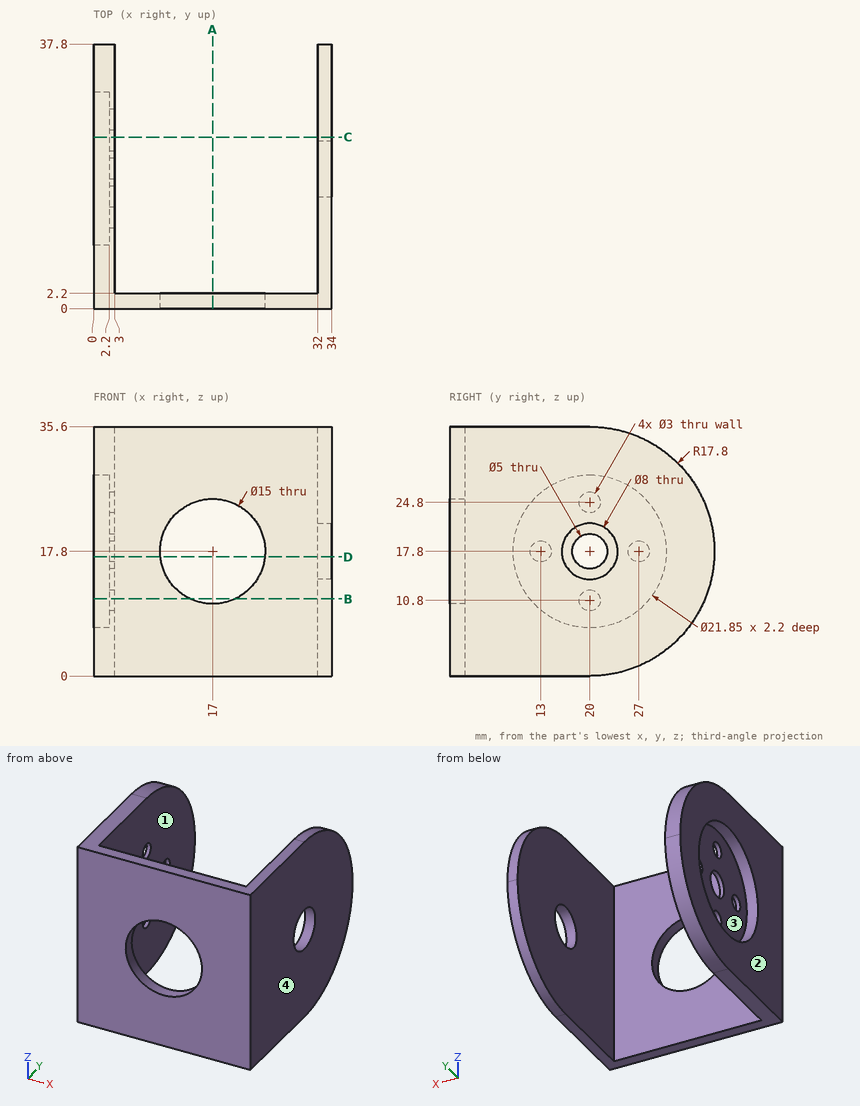
The figure shows three views and two pictorial views of one solid part (mm, origin at its lowest corner). Answer the questions. A direction names the side the tool comes from. Coordinates: 2 decimals unless noted, no trailing zeros. Loops run counter-clockwise (first coordinate to the right, second up) from the corner with the lowest first, then second, coordinate; pieces in that order, holes last. Notation, with made-up numbers: (25.25, 64.5) -> (73.25, 64.5) arc R22 ccw to (73.25, 96.5) -> close; hole circle Ø4 at (78.25, 65). An arc over 180 degrees is marked (long way). Return JSON: item names as keys, results as strings. Group by question number.
(1) Given pin 1 Ø3.5 at (y, z) = (27, 17.8) entering from -X; pin 2 Ø2.5 at (y, z) = (20, 10.8) entering from -X; pin 3 Ø7 at (y, z) = (20, 17.8) entering from +X; pin 4 Ø10 at (x, y) = (25, 22.5) entering from -Z, each flat-ended and moving along its own axis, determine where each tip first touches the part or whether it passes through.
(2) A cutting plane is placed at C-C on y = 24.5. Write down the section's boundary in (x, z).
(3) A cutting plane is placed at D-D on z = 17. Count the separate pieces of the cut face and the enclosed holes in it, and give its area (3 significant figures).
(4) Find the intervals of material crossed by probe 1 along X at (y, z) = (28, 7); probe 2 along Y at (x, z) = (32.6, 17.8); probe 3 along X at (y, z) = (28.5, 16.5), in increasing order. Write a range as from..to.
(5) A cutting plane is placed at B-B on z = 11. Write down the section's boundary in (x, y).
(6) Determine the mould class of the marked faces 3 and 4 for opening direction Z: released by +Z, released by -Z, zero draft, split by the parting line, or undercut.
(7) A cutting plane is placed at A-A on x = 17. Write down the section's boundary in (y, z), and give its area (3 significant figures).
(8) Which of the six approach directions +Z, -Z, +X, -X, +Y, -Y give full straight-line access (tool end or side, diameter ignored) to the marked faces 1 and 2?
The answers:
{
 "1": {"pin 1": "stops at x = 2.2", "pin 2": "stops at x = 32", "pin 3": "stops at x = 3", "pin 4": "passes through"},
 "2": {"outline": "(0, 0.58) -> (3, 0.58) -> (3, 35.02) -> (0, 35.02) -> (0, 27.76) -> (2.2, 27.76) -> (2.2, 7.84) -> (0, 7.84) -> close; (32, 0.58) -> (34, 0.58) -> (34, 35.02) -> (32, 35.02) -> close"},
 "3": {"separate pieces": "6", "enclosed holes": "0", "area": "148 mm^2"},
 "4": {"probe 1": "x = 0..3, 32..34", "probe 2": "y = 0..16, 24..37.8", "probe 3": "x = 2.2..3, 32..34"},
 "5": {"outline": "(0, 0) -> (13.84, 0) -> (13.84, 2.2) -> (3, 2.2) -> (3, 18.51) -> (2.2, 18.51) -> (2.2, 11.45) -> (0, 11.45) -> close; (0, 28.55) -> (2.2, 28.55) -> (2.2, 21.49) -> (3, 21.49) -> (3, 36.45) -> (0, 36.45) -> close; (20.16, 0) -> (34, 0) -> (34, 36.45) -> (32, 36.45) -> (32, 2.2) -> (20.16, 2.2) -> close"},
 "6": {"face 3": "undercut", "face 4": "zero draft"},
 "7": {"outline": "(0, 0) -> (2.2, 0) -> (2.2, 10.3) -> (0, 10.3) -> close; (0, 25.3) -> (2.2, 25.3) -> (2.2, 35.6) -> (0, 35.6) -> close", "area": "45.3 mm^2"},
 "8": {"face 1": "+Z, -Z, +Y", "face 2": "+Z, -Z, -X, +Y, -Y"}
}
